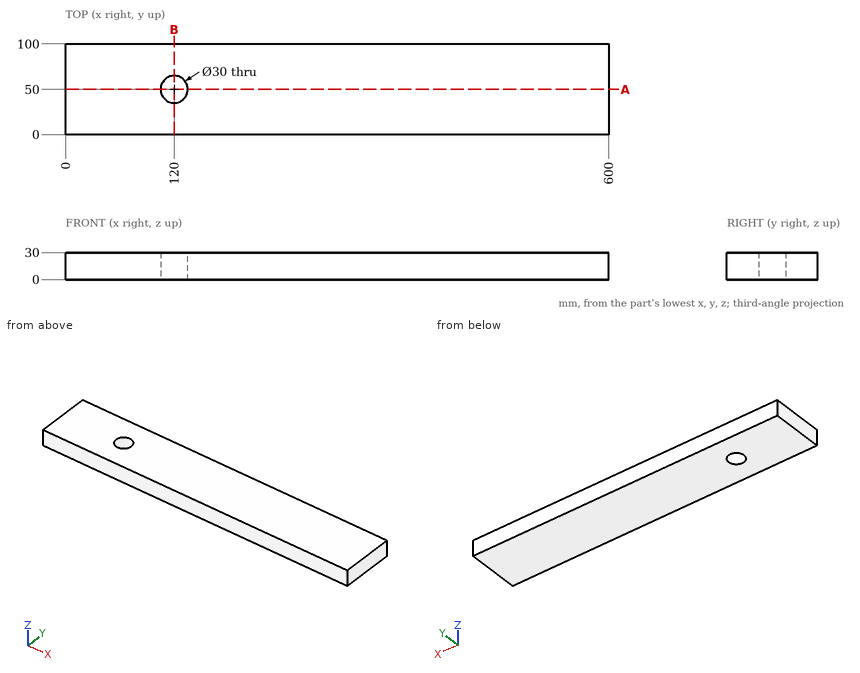
The drawing under review shows one solid part. Ordinate dimensions are in mm from its lowest x, y, z. Give positions to 0.01 mm unless a question says otherwise; leave off trailing zeros. Write each loop counter-clockwise with the first axis right and the second up, starting at its lowest first coordinate (ties: lowest second). Pieces come first, ordered by that corner, then holes. Notation, with made-up numbers: (70, -11) - (109, -11) arc R30 cw to (109, 24) - close; hole circle Ø3 at (84.25, 63.5). An arc over 180 degrees is marked (long way). Answer in a Markdown table with one row per item. Add a question column.
1. We need section B-B on x = 120. Write out the cut boundary in (y, z), then the cut area to 3 significant figures.
2. Wall thickness on line 1 along Y through (x, z) = (120, 8.5); line 2 along X through (y, z) = (51, 15); line 3 along X through (y, z) = (52, 3): over which ranges is each line inside the solid? List them lowest first. Write a range as [from, to].
3. Insertion check: P1, Ø3, axis at x = 234.5, z = 26.5, coming from the -Y side. The pin has a flat end and moves straight along its axis. Give the tip position at first contact, or say it passes through.
4. We need section A-A on y = 50. Write out the cut boundary in (x, z).
Ans:
| question | item | result |
|---|---|---|
| 1 | outline | (0, 0) - (35, 0) - (35, 30) - (0, 30) - close; (65, 0) - (100, 0) - (100, 30) - (65, 30) - close |
| 1 | area | 2,100 mm^2 |
| 2 | line 1 | y = [0, 35], [65, 100] |
| 2 | line 2 | x = [0, 105.03], [134.97, 600] |
| 2 | line 3 | x = [0, 105.13], [134.87, 600] |
| 3 | P1 | stops at y = 0 |
| 4 | outline | (0, 0) - (105, 0) - (105, 30) - (0, 30) - close; (135, 0) - (600, 0) - (600, 30) - (135, 30) - close |
